For this review, take the finished solid that the model builds, in its own axes (mm). Coordinates: 2 decimals unless noted, no trailing zeros. Order: outer loops, then holes, each group sorted by start corner. A loop starts at its lowest first (then second) coordinate and runs counter-clockwise, first axis right, second up. Notation, with made-up numbers: (55.25, 28) -> (113.25, 28) arc R7 ccw to (113.25, 35) -> close; hole circle Ø1 at (85, 72.5). An arc over 180 degrees is marked (long way). Write item = value, one per line. Start each with the question number.
1) Wall thickness on probe 1 along Z at (x, y) = (-118, 0.3); probe 2 along X at (y, z) = (1, -119.5); probe 3 along X at (y, z) = (0.7, 28): over which ranges is each line inside the solid? List them lowest first. Write a range as [from, to].
2) Consider section C-C on z = 42. Give the boundary of the cut face in (x, y), and give its area (3 significant figures).
3) Consider section A-A on x = -120. Give the boundary of the cut face in (y, z).
4) Consider section B-B on y = 1.3. Give the boundary of the cut face in (x, z), and give its area (3 significant figures).
5) Consider section D-D on z = 140. Give the boundary of the cut face in (x, y), and give its area (3 significant figures).
6) Insertion check: pin 1 Ø0.9 at (y, z) = (1, -123) entering from +X; pin 2 Ø0.9 at (y, z) = (2, -137.5) entering from +X; pin 3 Ø0.9 at (x, y) = (-268.5, 1.5) entering from -Z. Each pin has a flat end and moves straight along its axis. Give the tip position at first contact, or say it passes through.
from build123d import *

# Parameters (mm, degrees)
BOSS_EXTRUDE1_DEPTH = 3
SKETCH2_R           = 35
CUT_EXTRUDE1_DEPTH  = 3


with BuildPart() as part:
    # Sketch1 → Boss-Extrude1 (new body)
    with BuildSketch(Plane(origin=(0, 0, 0), x_dir=(1, 0, 0), z_dir=(0, 1, 0))):
        Polygon((-267, 136.567741935), (-240, 136.567741935), (-240, 139.567741935), (0, 139.567741935), (0, 136.567741935), (30, 136.567741935), (30, 106.567741935), (33, 106.567741935), (33, -133.432258065), (30, -133.432258065), (30, -163.432258065), (0, -163.432258065), (0, -166.432258065), (-240, -166.432258065), (-240, -163.432258065), (-267, -163.432258065), (-267, -133.432258065), (-270, -133.432258065), (-270, 106.567741935), (-267, 106.567741935), align=None)
    extrude(amount=BOSS_EXTRUDE1_DEPTH)

    # Sketch2 → Cut-Extrude1 (cut)
    with BuildSketch(Plane(origin=(0, 3, 0), x_dir=(1, 0, 0), z_dir=(0, 1, 0))):
        with Locations(Location((-120, -13.432258065, 0), (0, 0, 270))):
            Circle(SKETCH2_R)
    extrude(amount=-CUT_EXTRUDE1_DEPTH, mode=Mode.SUBTRACT)


solid = part.part
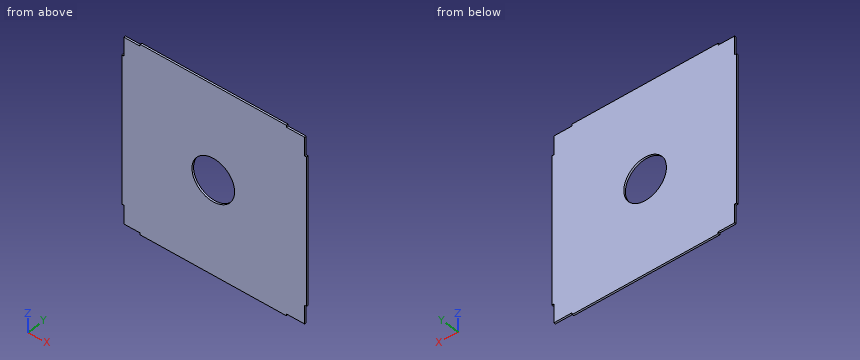
Answer sheet:
q1.probe_1 = [-139.57, -21.51], [48.38, 166.43]
q1.probe_2 = [-267, 30]
q1.probe_3 = [-270, -151.82], [-88.18, 33]
q2.outline = (-270, 0) -> (-140.22, 0) -> (-140.22, 3) -> (-270, 3) -> close; (-99.78, 0) -> (33, 0) -> (33, 3) -> (-99.78, 3) -> close
q2.area = 788 mm2
q3.outline = (0, -139.57) -> (3, -139.57) -> (3, -21.57) -> (0, -21.57) -> close; (0, 48.43) -> (3, 48.43) -> (3, 166.43) -> (0, 166.43) -> close
q4.outline = (-270, -106.57) -> (-267, -106.57) -> (-267, -136.57) -> (-240, -136.57) -> (-240, -139.57) -> (0, -139.57) -> (0, -136.57) -> (30, -136.57) -> (30, -106.57) -> (33, -106.57) -> (33, 133.43) -> (30, 133.43) -> (30, 163.43) -> (0, 163.43) -> (0, 166.43) -> (-240, 166.43) -> (-240, 163.43) -> (-267, 163.43) -> (-267, 133.43) -> (-270, 133.43) -> close; hole circle Ø70 at (-120, 13.43)
q4.area = 88,100 mm2
q5.outline = (-267, 0) -> (30, 0) -> (30, 3) -> (-267, 3) -> close
q5.area = 891 mm2
q6.pin_1 = 30
q6.pin_2 = 0
q6.pin_3 = -106.57
